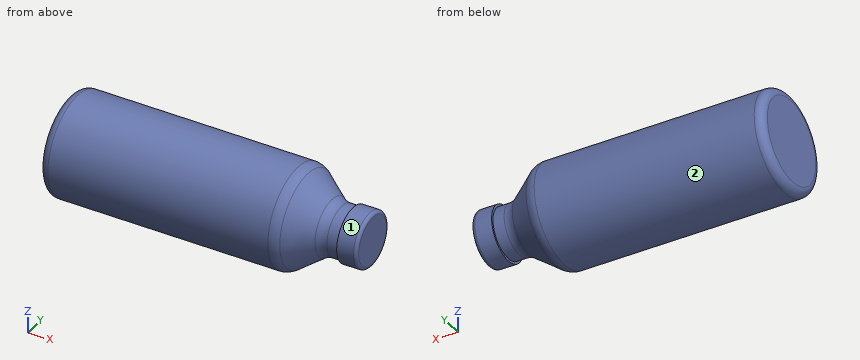
from build123d import *

# Parameters (mm, degrees)
FILLET_1_R      = 5
SHELL_1_T       = -1
EXTRUDE_START   = -10
SKETCH_2_R      = 16.391613339
SKETCH_2_R_2    = 15
EXTRUDE_1_DEPTH = 10
SKETCH_3_R      = 16.391613339
EXTRUDE_2_DEPTH = 2
FILLET_2_R      = 2


with BuildPart() as part:
    # 草图1 → 旋转1 (revolve)
    with BuildSketch(Plane.XY, mode=Mode.PRIVATE) as revolve_1_sk:
        with BuildLine():
            Line((180, 15), (163.333333333, 15))
            ThreePointArc((163.333333333, 15), (160.171055673, 15.513167019), (157.333333333, 17))
            Line((157.333333333, 17), (142.666666667, 28))
            ThreePointArc((142.666666667, 28), (139.828944327, 29.486832981), (136.666666667, 30))
            Line((136.666666667, 30), (0, 30))
            Line((0, 30), (0, 0))
            Line((0, 0), (180, 0))
            Line((180, 0), (180, 15))
        make_face()
    revolve(revolve_1_sk.sketch.rotate(Axis((0, 0, 0), (1, 0, 0)), 90), axis=Axis((0, 0, 0), (1, 0, 0)))

    # 圆角1
    fillet_1_edges = [part.edges().sort_by_distance(p)[0] for p in [
        (0, 0, -30),
    ]]
    fillet(fillet_1_edges, radius=FILLET_1_R)

    # 抽壳1
    shell_1_openings = [part.faces().sort_by_distance(p)[0] for p in [
        (180, 0, 0),
    ]]
    offset(amount=SHELL_1_T, openings=shell_1_openings, kind=Kind.INTERSECTION)

    # 草图2 → 凸台-拉伸1 (add)
    with BuildSketch(Plane(origin=(180, 0, 0), x_dir=(0, 0, -1), z_dir=(1, 0, 0)).offset(EXTRUDE_START)):
        Circle(SKETCH_2_R)
        with Locations(Location((0, 0, 0), (0, 0, 180))):
            Circle(SKETCH_2_R_2, mode=Mode.SUBTRACT)
    extrude(amount=EXTRUDE_1_DEPTH)

    # 草图3 → 凸台-拉伸2 (add)
    with BuildSketch(Plane(origin=(180, 0, 0), x_dir=(0, 0, -1), z_dir=(1, 0, 0))):
        Circle(SKETCH_3_R)
    extrude(amount=EXTRUDE_2_DEPTH)

    # 圆角2
    fillet_2_edges = [part.edges().sort_by_distance(p)[0] for p in [
        (182, 0, 16.391613339),
    ]]
    fillet(fillet_2_edges, radius=FILLET_2_R)


solid = part.part
Geometry check sheet. Reference: the model listing, model coordinates, mm. Face numbers are marked on the shaded views. A direction names the side the tool comes from. Give positions to 0.01 mm unless a question says otherwise; leave off trailing zeros. Order: outer loops, then holes, each group sorted by start corner. A loop starts at its lowest first (then second) coordinate and runs counter-clockwise, first axis right, second up.
1) Material ranges on probe 1 along Y at (x, z) = (89, 0); probe 2 along Y at (x, z) = (171.75, 0); probe 3 along X at (y, z) = (-11, 2.5), recorded low to high.
Results are:
probe 1: y = -30 to -29, 29 to 30
probe 2: y = -16.39 to -14, 14 to 16.39
probe 3: x = 0 to 1, 180 to 182
2) Gauge pin test, flat ends, axial feed: pin 1 (3 mm diameter, centred on x = 86.5, y = -3, fed in from +Z); pin 2 (6 mm diameter, centred on x = 58, z = 20, fed in from -Y); pin 3 (12 mm diameter, centred on x = 124, y = -13, fed in from +Z). Record the tip position at first contact, or that the pin passes through.
Results are:
pin 1: stops at z = 29.96
pin 2: stops at y = -24.72
pin 3: stops at z = 29.17
3) Cross-section at C-C (x = 121.5). Record the boundary of the cut face in (y, z).
Results are:
outline: circle Ø60 at (0, 0); hole circle Ø58 at (0, 0)
4) Tool access check on the marked faces 1 and 2. Record the directions out of +Z, -Z, +X, -X, +Y, -Y that give a thin tool (end or side, any length) a straight path to the whole face; none if there is none.
Results are:
face 1: +X
face 2: +X, -X
